from build123d import *

# Parameters (mm, degrees)
F0_W     = 15
F0_H     = 8
F1_DEPTH = 15
F1_TAPER = 3
F2_R     = 2.5
F3_DEPTH = 5
F4_R     = 1


with BuildPart() as f1:
    # F0 (on Top) → F1 (new body)
    with BuildSketch(Plane.XY):
        Rectangle(F0_W, F0_H)
    extrude(amount=F1_DEPTH, taper=F1_TAPER)

    # F2 (on face) → F3 (join)
    with BuildSketch(Plane.XY.offset(15)):
        Circle(F2_R)
    extrude(amount=F3_DEPTH)

    # F4
    f4_edges = [f1.edges().sort_by_distance(p)[0] for p in [
        (-7.106942, -3.606942, 7.5),
        (7.106942, -3.606942, 7.5),
        (7.106942, 3.606942, 7.5),
        (6.713883, 0, 15),
        (0, -3.213883, 15),
        (-6.713883, 0, 15),
        (0, 3.213883, 15),
        (-7.106942, 3.606942, 7.5),
    ]]
    fillet(f4_edges, radius=F4_R)


solid = f1.part
Input: part model. Units: mm. Frame: model coordinates. A direction names the side the tool comes from. Give positions to 0.01 mm unless a question says otherwise; leave off trailing zeros. Write each loop counter-clockwise with the first axis right and the second up, starting at its lowest first coordinate (ties: lowest second). Pieces come first, ordered by that corner, then holes. Notation, with made-up numbers: (59.25, 36) -> (78.25, 36) arc R18 ccw to (78.25, 71) -> close; hole circle Ø1 at (36.25, 45.5). An arc over 180 degrees is marked (long way). Use one line per item in the form item = value. Start each with the question number.
1) Set-up query: faces 4 (the flat face through (0, 0, 20)), 5 (the cylindrical face through (3.38, 2.96, 14.72)), 6 (the cylindrical face through (-0.54, -2.44, 17.46)), 7 (the cylindrical face through (-3.38, -2.96, 14.72)). Return all of +Z, -Z, +X, -X, +Y, -Y with unobstructed straight access to the full face (end or side cutting, diameter ignored); none if empty.
2) Section query C-C on z = 15.5. Return the cut outline in (x, y), then the cut area to 3 significant figures.
3) Section query B-B on x = 2. Return the cut outline in (y, z).
4) Pin query (flat end, axial travel): pin 1 (3 mm diameter, centred on y = 1.5, z = 14, fed in from +X); pin 2 (5 mm diameter, centred on x = 5, z = 10, fed in from +Y); pin 3 (3 mm diameter, centred on y = 1.5, z = 8, fed in from +X). Return the tip coordinate at first contact, or that it passes through.
5) Ray query, probe 1 along Z at (x, y) = (5.5, 0); probe 2 along Y at (x, z) = (-1.5, 14); probe 3 along X at (y, z) = (1.5, 6.5). Return the intervals inside material, ascending. Write a range as from..to.
6) Draft query along Y for faces 1 (the cylindrical face through (3.44, -2.96, 14.72)), 2 (the flat face through (-0.091, 3.636, 6.947)), 3 (the cylindrical face through (-6.46, -0.03, 14.72)). Return one class per face: pulls with the +Y half, pulls with the -Y half, needs draft (parallel to the pull), parting line crosses it, or undercut.
7) Section query A-A on y = 0. Return the cut outline in (x, z), then the cut area to 3 significant figures.
Outcome:
q1.face_4 = +Z, +X, -X, +Y, -Y
q1.face_5 = +Z, +X, +Y
q1.face_6 = +Z
q1.face_7 = +Z, -X, -Y
q2.outline = circle Ø5 at (0, 0)
q2.area = 19.6 mm^2
q3.outline = (-4, 0) -> (4, 0) -> (3.26, 14.05) arc R1 ccw to (2.26, 15) -> (1.5, 15) -> (1.5, 20) -> (-1.5, 20) -> (-1.5, 15) -> (-2.26, 15) arc R1 ccw to (-3.26, 14.05) -> close
q4.pin_1 = 6.84
q4.pin_2 = 3.61
q4.pin_3 = 7.16
q5.probe_1 = 0..15
q5.probe_2 = -3.27..3.27
q5.probe_3 = -7.16..7.16
q6.face_1 = pulls with the -Y half
q6.face_2 = pulls with the +Y half
q6.face_3 = needs draft
q7.outline = (-7.5, 0) -> (7.5, 0) -> (6.76, 14.05) arc R1 ccw to (5.76, 15) -> (2.5, 15) -> (2.5, 20) -> (-2.5, 20) -> (-2.5, 15) -> (-5.76, 15) arc R1 ccw to (-6.76, 14.05) -> close
q7.area = 238 mm^2
